For this review, take the finished solid that the model builds, in its own axes (mm). A direction names the side the tool comes from. Round coordinates to 2 decimals unless told otherwise and drop trailing zeros. Order: outer loops, then holes, each group sorted by start corner. A loop starts at its lowest first (then second) coordinate and runs counter-clockwise, first axis right, second up.
from build123d import *

# Parameters (mm, degrees)
SKETCH_1_W          = 36
SKETCH_1_H          = 30
EXTRUDE_1_DEPTH     = 3
SKETCH_3_R          = 3
EXTRUDE_2_DEPTH     = 2
SKETCH_4_W          = 5
SKETCH_4_H          = 9
CUT_EXTRUDE_2_DEPTH = 47.957427527
HOLE_WIZARD_M6_1_D  = 5
FILLET_1_R          = 0.5
MM_1_D              = 2.5
FILLET_2_R          = 2


with BuildPart() as part:
    # 草图1 → 凸台-拉伸1 (new body)
    with BuildSketch(Plane.XY):
        with Locations((18, 15)):
            Rectangle(SKETCH_1_W, SKETCH_1_H)
    extrude(amount=EXTRUDE_1_DEPTH)

    # 草图3 → 凸台-拉伸2 (add)
    with BuildSketch(Plane.XY.offset(3)):
        with Locations(Location((8, 23, 0), (0, 0, 180))):
            Circle(SKETCH_3_R)
        with Locations(Location((8, 7, 0), (0, 0, 180))):
            Circle(SKETCH_3_R)
        with Locations(Location((28, 7, 0), (0, 0, 180))):
            Circle(SKETCH_3_R)
        with Locations(Location((28, 23, 0), (0, 0, 180))):
            Circle(SKETCH_3_R)
    extrude(amount=EXTRUDE_2_DEPTH)

    # 草图4 → 切除-拉伸2 (cut, through all)
    with BuildSketch(Plane.XY.offset(3)):
        with Locations((33.5, 15)):
            Rectangle(SKETCH_4_W, SKETCH_4_H)
        with Locations((2.5, 15)):
            Rectangle(SKETCH_4_W, SKETCH_4_H)
    extrude(amount=-CUT_EXTRUDE_2_DEPTH, mode=Mode.SUBTRACT)

    # M6 螺纹孔1 (through all)
    with Locations(Plane(origin=(18, 15, 3), x_dir=(1, 0, 0), z_dir=(0, 0, 1))):
        with Locations((0, 0)):
            Hole(HOLE_WIZARD_M6_1_D / 2)

    # 圆角1
    fillet_1_edges = [part.edges().sort_by_distance(p)[0] for p in [
        (5, 19.5, 1.5),
        (5, 10.5, 1.5),
        (31, 10.5, 1.5),
        (31, 19.5, 1.5),
    ]]
    fillet(fillet_1_edges, radius=FILLET_1_R)

    # 大小mm 暗销孔1 (through all)
    with Locations(Plane(origin=(3, 27, 3), x_dir=(1, 0, 0), z_dir=(0, 0, 1))):
        with Locations((0, 0), (10, 0), (20, 0), (30, 0), (30, -24), (20, -24), (10, -24), (0, -24)):
            Hole(MM_1_D / 2)

    # 圆角2
    fillet_2_edges = [part.edges().sort_by_distance(p)[0] for p in [
        (0, 30, 1.5),
        (36, 30, 1.5),
        (36, 0, 1.5),
        (0, 0, 1.5),
    ]]
    fillet(fillet_2_edges, radius=FILLET_2_R)


solid = part.part
(1) Tool access review of faces 4 (the face through (5, 15, 2)), 5 (the face through (31, 23, 4)), 6 (the face through (13.921, 27.845, 1.479)), 7 (the face through (34, 10.5, 2)): name each direction out of +Z, -Z, +X, -X, +Y, -Y from which nothing blocks a thin tool from reaching the whole face with its end or side.
(2) Add section B-B on x = 16.5. Give the boundary of the cut face in (y, z).
(3) Wall thickness on L1, parallel to Y at x = 33, z = 1.85; L2, parallel to Y at x = 13, z = 1.6; L3, parallel to Y at x = 18, z = 1.05: over which ranges is each line inside the solid? List them lowest first.
(4) Draft analysis for pull direction Y (two halves, no side actions). For faces 1 (the face through (35.4, 29.43, 1.52)), 2 (the face through (2, 10.5, 2)), 3 (the face through (28, 23, 5)), state which applies: pulls with the +Y half, pulls with the -Y half, needs draft (parallel to the pull), parting line crosses it, or undercut.
(5) Add section C-C on x = 33. Give the boundary of the cut face in (y, z).
(6) Add section A-A on y = 13.5. Give the boundary of the cut face in (x, z).
(7) Clearance check with flat-ended pins moving along their axes: P1, Ø2, axis at x = 23, y = 3, coming from the -Z side; P2, Ø4, axis at x = 18.5, y = 13.5, coming from the +Z side; P3, Ø1.5, axis at y = 20.5, z = 4.5, coming from the +X side; P4, Ø1, axis at x = 27.5, z = 4, coming from the -Y side. State where each tip first meets the part, or that it passes through.
(8) Add section D-D on y = 3. Give the boundary of the cut face in (x, z).
Here are the results:
1. face 4: +Z, -Z, -X
1. face 5: +Z
1. face 6: +Z, -Z
1. face 7: +Z, -Z, +X
2. outline: (0, 0) - (13, 0) - (13, 3) - (0, 3) - close; (17, 0) - (30, 0) - (30, 3) - (17, 3) - close
3. L1: y = 0 to 1.75, 4.25 to 10.5, 19.5 to 25.75, 28.25 to 30
3. L2: y = 0 to 1.75, 4.25 to 25.75, 28.25 to 30
3. L3: y = 0 to 12.5, 17.5 to 30
4. face 1: pulls with the +Y half
4. face 2: undercut
4. face 3: needs draft
5. outline: (0, 0) - (1.75, 0) - (1.75, 3) - (0, 3) - close; (4.25, 0) - (10.5, 0) - (10.5, 3) - (4.25, 3) - close; (19.5, 0) - (25.75, 0) - (25.75, 3) - (19.5, 3) - close; (28.25, 0) - (30, 0) - (30, 3) - (28.25, 3) - close
6. outline: (5, 0) - (16, 0) - (16, 3) - (5, 3) - close; (20, 0) - (31, 0) - (31, 3) - (20, 3) - close
7. P1: passes through
7. P2: stops at z = 3
7. P3: stops at x = 30.44
7. P4: stops at y = 4
8. outline: (0, 0) - (1.75, 0) - (1.75, 3) - (0, 3) - close; (4.25, 0) - (11.75, 0) - (11.75, 3) - (4.25, 3) - close; (14.25, 0) - (21.75, 0) - (21.75, 3) - (14.25, 3) - close; (24.25, 0) - (31.75, 0) - (31.75, 3) - (24.25, 3) - close; (34.25, 0) - (36, 0) - (36, 3) - (34.25, 3) - close
